from build123d import *

# Parameters (mm, degrees)
CYLINDER_R         = 1.5
CYLINDER_DEPTH     = 10
BOX014_W           = 2.54
BOX014_H           = 10
BOX014_DEPTH       = 2.54
BOX013_W           = 2.53
BOX013_H           = 10
BOX013_DEPTH       = 2.53
BOX012_W           = 2.54
BOX012_H           = 10.16
BOX012_DEPTH       = 2.6
BOX011_W           = 0.64
BOX011_H           = 0.64
BOX011_DEPTH       = 9.9
BOX011_PITCH_ANGLE = 90
BOX010_W           = 0.64
BOX010_H           = 0.64
BOX010_DEPTH       = 9.9
BOX009_W           = 0.64
BOX009_H           = 0.64
BOX009_DEPTH       = 9.9
BOX009_PITCH_ANGLE = 90
BOX008_W           = 0.64
BOX008_H           = 0.64
BOX008_DEPTH       = 9.9
BOX007_W           = 0.64
BOX007_H           = 0.64
BOX007_DEPTH       = 9.9
BOX007_PITCH_ANGLE = 90
BOX006_W           = 0.64
BOX006_H           = 0.64
BOX006_DEPTH       = 9.9
BOX005_W           = 0.64
BOX005_H           = 0.64
BOX005_DEPTH       = 9.9
BOX005_PITCH_ANGLE = 90
BOX004_W           = 0.64
BOX004_H           = 0.64
BOX004_DEPTH       = 9.9
FILLET_R           = 0.4
FILLET001_R        = 0.4
FILLET002_R        = 0.4
FILLET003_R        = 0.4
FILLET004_R        = 0.4
FILLET005_R        = 0.4
FILLET006_R        = 0.4
FILLET007_R        = 0.4
BOX003_W           = 6
BOX003_H           = 5
BOX003_DEPTH       = 3.25
BOX002_W           = 6
BOX002_H           = 4.5
BOX002_DEPTH       = 11.5
BOX001_W           = 6
BOX001_H           = 4.5
BOX001_DEPTH       = 11.5
BOX_W              = 32
BOX_H              = 14.05
BOX_DEPTH          = 1.2


with BuildPart() as cylinder:
    # Cylinder → Cylinder (new body)
    with BuildSketch(Plane(origin=(7.75, 7, 0), x_dir=(1, 0, 0), z_dir=(0, 0, 1))):
        Circle(CYLINDER_R)
    extrude(amount=CYLINDER_DEPTH)


with BuildPart() as box014:
    # Box014 → Box014 (new body)
    with BuildSketch(Plane(origin=(-0.5, -1, 0), x_dir=(1, 0, 0), z_dir=(0, 0, 1))):
        with Locations((1.27, 5)):
            Rectangle(BOX014_W, BOX014_H)
    extrude(amount=BOX014_DEPTH)


with BuildPart() as box013:
    # Box013 → Box013 (new body)
    with BuildSketch(Plane(origin=(-9.9, -1, 8.9), x_dir=(1, 0, 0), z_dir=(0, 0, 1))):
        with Locations((1.265, 5)):
            Rectangle(BOX013_W, BOX013_H)
    extrude(amount=BOX013_DEPTH)


with BuildPart() as box012:
    # Box012 → Box012 (new body)
    with BuildSketch(Plane(origin=(-0.95, -0.95, 5.69), x_dir=(1, 0, 0), z_dir=(0, 0, 1))):
        with Locations((1.27, 5.08)):
            Rectangle(BOX012_W, BOX012_H)
    extrude(amount=BOX012_DEPTH)


with BuildPart() as box011:
    # Box011 → Box011 (new body)
    with BuildSketch(Plane.XY):
        with Locations((0.32, 0.32)):
            Rectangle(BOX011_W, BOX011_H)
    extrude(amount=BOX011_DEPTH)


with BuildPart() as box011_1:
    # Box011 pitch: moved
    add(box011.part.rotate(Axis((0, 0, 0), (0, 1, 0)), BOX011_PITCH_ANGLE))


with BuildPart() as box011_2:
    # Box011 placement: moved
    add(box011_1.part.moved(Location((-9.9, 7.62, 9.9))))


with BuildPart() as box010:
    # Box010 → Box010 (new body)
    with BuildSketch(Plane(origin=(0, 7.62, 0), x_dir=(1, 0, 0), z_dir=(0, 0, 1))):
        with Locations((0.32, 0.32)):
            Rectangle(BOX010_W, BOX010_H)
    extrude(amount=BOX010_DEPTH)


with BuildPart() as box009:
    # Box009 → Box009 (new body)
    with BuildSketch(Plane.XY):
        with Locations((0.32, 0.32)):
            Rectangle(BOX009_W, BOX009_H)
    extrude(amount=BOX009_DEPTH)


with BuildPart() as box009_1:
    # Box009 pitch: moved
    add(box009.part.rotate(Axis((0, 0, 0), (0, 1, 0)), BOX009_PITCH_ANGLE))


with BuildPart() as box009_2:
    # Box009 placement: moved
    add(box009_1.part.moved(Location((-9.9, 5.08, 9.9))))


with BuildPart() as box008:
    # Box008 → Box008 (new body)
    with BuildSketch(Plane(origin=(0, 5.08, 0), x_dir=(1, 0, 0), z_dir=(0, 0, 1))):
        with Locations((0.32, 0.32)):
            Rectangle(BOX008_W, BOX008_H)
    extrude(amount=BOX008_DEPTH)


with BuildPart() as box007:
    # Box007 → Box007 (new body)
    with BuildSketch(Plane.XY):
        with Locations((0.32, 0.32)):
            Rectangle(BOX007_W, BOX007_H)
    extrude(amount=BOX007_DEPTH)


with BuildPart() as box007_1:
    # Box007 pitch: moved
    add(box007.part.rotate(Axis((0, 0, 0), (0, 1, 0)), BOX007_PITCH_ANGLE))


with BuildPart() as box007_2:
    # Box007 placement: moved
    add(box007_1.part.moved(Location((-9.9, 2.54, 9.9))))


with BuildPart() as box006:
    # Box006 → Box006 (new body)
    with BuildSketch(Plane(origin=(0, 2.54, 0), x_dir=(1, 0, 0), z_dir=(0, 0, 1))):
        with Locations((0.32, 0.32)):
            Rectangle(BOX006_W, BOX006_H)
    extrude(amount=BOX006_DEPTH)


with BuildPart() as box005:
    # Box005 → Box005 (new body)
    with BuildSketch(Plane.XY):
        with Locations((0.32, 0.32)):
            Rectangle(BOX005_W, BOX005_H)
    extrude(amount=BOX005_DEPTH)


with BuildPart() as box005_1:
    # Box005 pitch: moved
    add(box005.part.rotate(Axis((0, 0, 0), (0, 1, 0)), BOX005_PITCH_ANGLE))


with BuildPart() as box005_2:
    # Box005 placement: moved
    add(box005_1.part.moved(Location((-9.9, 0, 9.9))))


with BuildPart() as cut001:
    # Box004 → Box004 (new body)
    with BuildSketch(Plane.XY):
        with Locations((0.32, 0.32)):
            Rectangle(BOX004_W, BOX004_H)
    extrude(amount=BOX004_DEPTH)

    # Fusion003: union Box005
    add(box005_2.part)

    # Fusion004: union Box006
    add(box006.part)

    # Fusion005: union Box007
    add(box007_2.part)

    # Fusion006: union Box008
    add(box008.part)

    # Fusion007: union Box009
    add(box009_2.part)

    # Fusion008: union Box010
    add(box010.part)

    # Fusion009: union Box011
    add(box011_2.part)

    # Fusion010: union Box012
    add(box012.part)

    # Fillet
    fillet_edges = [cut001.edges().sort_by_distance(p)[0] for p in [
        (0.64, 0.32, 9.9),
    ]]
    fillet(fillet_edges, radius=FILLET_R)

    # Fillet001
    fillet001_edges = [cut001.edges().sort_by_distance(p)[0] for p in [
        (0.64, 2.86, 9.9),
    ]]
    fillet(fillet001_edges, radius=FILLET001_R)

    # Fillet002
    fillet002_edges = [cut001.edges().sort_by_distance(p)[0] for p in [
        (0.64, 5.4, 9.9),
    ]]
    fillet(fillet002_edges, radius=FILLET002_R)

    # Fillet003
    fillet003_edges = [cut001.edges().sort_by_distance(p)[0] for p in [
        (0.64, 7.94, 9.9),
    ]]
    fillet(fillet003_edges, radius=FILLET003_R)

    # Fillet004
    fillet004_edges = [cut001.edges().sort_by_distance(p)[0] for p in [
        (0, 7.94, 9.26),
    ]]
    fillet(fillet004_edges, radius=FILLET004_R)

    # Fillet005
    fillet005_edges = [cut001.edges().sort_by_distance(p)[0] for p in [
        (0, 5.4, 9.26),
    ]]
    fillet(fillet005_edges, radius=FILLET005_R)

    # Fillet006
    fillet006_edges = [cut001.edges().sort_by_distance(p)[0] for p in [
        (0, 2.86, 9.26),
    ]]
    fillet(fillet006_edges, radius=FILLET006_R)

    # Fillet007
    fillet007_edges = [cut001.edges().sort_by_distance(p)[0] for p in [
        (0, 0.32, 9.26),
    ]]
    fillet(fillet007_edges, radius=FILLET007_R)

    # Cut: cut Box013
    add(box013.part, mode=Mode.SUBTRACT)

    # Cut001: cut Box014
    add(box014.part, mode=Mode.SUBTRACT)


with BuildPart() as cut001_1:
    # Cut001 placement: moved
    add(cut001.part.moved(Location((2, 3, -4.5))))


with BuildPart() as box003:
    # Box003 → Box003 (new body)
    with BuildSketch(Plane(origin=(26, 4.5, 0), x_dir=(1, 0, 0), z_dir=(0, 0, 1))):
        with Locations((3, 2.5)):
            Rectangle(BOX003_W, BOX003_H)
    extrude(amount=BOX003_DEPTH)


with BuildPart() as box002:
    # Box002 → Box002 (new body)
    with BuildSketch(Plane(origin=(26, 0, 0), x_dir=(1, 0, 0), z_dir=(0, 0, 1))):
        with Locations((3, 2.25)):
            Rectangle(BOX002_W, BOX002_H)
    extrude(amount=BOX002_DEPTH)


with BuildPart() as box001:
    # Box001 → Box001 (new body)
    with BuildSketch(Plane(origin=(26, 9.5, 0), x_dir=(1, 0, 0), z_dir=(0, 0, 1))):
        with Locations((3, 2.25)):
            Rectangle(BOX001_W, BOX001_H)
    extrude(amount=BOX001_DEPTH)


with BuildPart() as cut002:
    # Box → Box (new body)
    with BuildSketch(Plane.XY):
        with Locations((16, 7.025)):
            Rectangle(BOX_W, BOX_H)
    extrude(amount=BOX_DEPTH)

    # Fusion: union Box001
    add(box001.part)

    # Fusion001: union Box002
    add(box002.part)

    # Fusion002: union Box003
    add(box003.part)

    # Fusion011: union Cut001
    add(cut001_1.part)

    # Cut002: cut Cylinder
    add(cylinder.part, mode=Mode.SUBTRACT)


solid = cut002.part
Could you check a few things on this model? Use its own coordinates, in mm. A direction names the side the tool comes from. Give positions to 0.01 mm unless a question says otherwise; leave off trailing zeros. Write each loop counter-clockwise with the first axis right and the second up, starting at its lowest first coordinate (ties: lowest second). Pieces come first, ordered by that corner, then holes. Notation, with made-up numbers: (60.5, 36) -> (65.5, 36) arc R20 ccw to (65.5, 63) -> close; hole circle Ø10 at (-10.75, 37.5). An arc over 180 degrees is marked (long way). Write each question's results on one line, items separated by ' | '. Start each with the question number.
Q1. I need wall thicknesses on probe 1 along Y at (x, z) = (-4, 5); probe 2 along Y at (x, z) = (7.75, 0.4); probe 3 along X at (y, z) = (7, 0.95). Which ranges of each line are inside material? Lowest first, please.
Q2. Suppose I cut it at D-D, the plane x = -0.5. List the corners of the cut face in (y, z) for me.
Q3. Suppose I cut it at A-A, the plane z = 9. List the corners of the cut face in (x, y) for me, and give its area (3 significant figures).
Q4. I'm going to push flat-ended pins straight in: pin 1 Ø0.5 at (y, z) = (11, -1) entering from -X; pin 2 Ø1.8 at (x, z) = (-1.5, 5) entering from -Y; pin 3 Ø5 at (x, y) = (21, 12.5) entering from -Z. Where does each tip first touch, or does it pass through?
Q5. Which directions (+Z, -Z, +X, -X, +Y, -Y) give clear straight access to the entire face, cutting with the end or side of a thin tool? Please do faces 1 (the face through (2, 12.21, 2)), 2 (the face through (-1, 5.54, 5)), 3 (the face through (-1, 3.64, 5)).
Q6. We'd pull the mould along X, two halves only. Please class faces 4 (the face through (6.56, 6.09, 0.59)), 5 (the face through (26, 7, 3)), 6 (the face through (-1, 8.08, 5)): +X half, -X half, draft (parallel to the pull), parting line (faces both ways), or undercut.
Q7. Suppose I cut it at C-C, the plane y = 7. List the corners of the cut face in (x, z) for me.
Q8. Suppose I cut it at B-B, the plane x = 7.75. List the corners of the cut face in (y, z) for me, and give its area (3 significant figures).
Outcome:
1) probe 1: 3 to 3.64, 5.54 to 6.18, 8.08 to 8.72, 10.62 to 11.26 | probe 2: 0 to 5.5, 8.5 to 14.05 | probe 3: 0 to 6.25, 9.25 to 32
2) outline: (3, 4.76) -> (3.64, 4.76) -> (3.64, 5.4) -> (3, 5.4) -> close; (5.54, 4.76) -> (6.18, 4.76) -> (6.18, 5.4) -> (5.54, 5.4) -> close; (8.08, 4.76) -> (8.72, 4.76) -> (8.72, 5.4) -> (8.08, 5.4) -> close; (10.62, 4.76) -> (11.26, 4.76) -> (11.26, 5.4) -> (10.62, 5.4) -> close
3) outline: (26, 0) -> (32, 0) -> (32, 4.5) -> (26, 4.5) -> close; (26, 9.5) -> (32, 9.5) -> (32, 14) -> (26, 14) -> close | area: 54.0 mm2
4) pin 1: x = 2 | pin 2: y = 3 | pin 3: z = 0
5) face 1: +Z, -X, +Y | face 2: +Z, +X, -X | face 3: +Z, -X
6) face 4: undercut | face 5: undercut | face 6: draft
7) outline: (0, 0) -> (6.25, 0) -> (6.25, 1.2) -> (3.59, 1.2) -> (3.59, 3.79) -> (1.05, 3.79) -> (1.05, 1.2) -> (0, 1.2) -> close; (9.25, 0) -> (32, 0) -> (32, 3.25) -> (26, 3.25) -> (26, 1.2) -> (9.25, 1.2) -> close
8) outline: (0, 0) -> (5.5, 0) -> (5.5, 1.2) -> (0, 1.2) -> close; (8.5, 0) -> (14.05, 0) -> (14.05, 1.2) -> (8.5, 1.2) -> close | area: 13.3 mm2
